Geometry: final body of the model. Coordinates: model frame, mm. Give positions to 0.01 mm unless a question says otherwise; leave off trailing zeros. Order: outer loops, then holes, each group sorted by start corner. A loop starts at its lowest first (then second) coordinate and runs counter-clockwise, first axis right, second up. Notation, with made-up numbers: M 21.25,72.5 L 78.25,72.5 A34 ccw 78.25,111.5 Z; hole C 48.25,-34 d6. An arc over 180 degrees is marked long. Write item = value, one per line. Start each with the question number.
from build123d import *

# Parameters (mm, degrees)
F1_ANGLE    = 180
F2_R        = 3.75
F3_DEPTH    = 5
F4_T4_ANGLE = 81.9757587875


# Not quite as in the source:
# - a fillet or chamfer that OpenCascade refuses, or shapes differently, is made with other operations: its cross-section is extruded or revolved along the edge and cut away or added
# - a feature names something its author has since deleted; it is built from what else it names


with BuildPart() as f1:
    # F0 (on Top) → F1 (revolve)
    with BuildSketch(Plane.XY):
        with BuildLine():
            ThreePointArc((-26, 0), (0, 26), (26, 0))
            Line((26, 0), (28.5, 0))
            ThreePointArc((28.5, 0), (0, 28.5), (-28.5, 0))
            Line((-28.5, 0), (-26, 0))
        make_face()
    revolve(axis=Axis((0, 0, 0), (1, 0, 0)), revolution_arc=F1_ANGLE)

    # F2 (on Top) → F3 (join)
    with BuildSketch(Plane.XY):
        with BuildLine():
            Line((64.7386337537, 8), (24.7386337537, 8))
            ThreePointArc((24.7386337537, 8), (25.6827225737, 4.0494149209), (26, 0))
            ThreePointArc((26, 0), (25.6827225737, -4.0494149209), (24.7386337537, -8))
            Line((24.7386337537, -8), (66.83281573, -8))
            ThreePointArc((66.83281573, -8), (72.8068677326, 0.918971944), (64.7386337537, 8))
        make_face()
        with Locations((64.7386337537, -0.1370499422)):
            Circle(F2_R, mode=Mode.SUBTRACT)
    extrude(amount=F3_DEPTH)

    # F4: chamfer of 5 on 1 edges, made by hand


with BuildPart() as f4_tool2:
    # F4_s3 → F4_t4 (revolve)
    with BuildSketch(Plane(origin=(0, 0, 0), x_dir=(0, 0, 1), z_dir=(-0.6558993597, -0.754848349, 0))):
        with BuildLine():
            Line((4.8832304356, -32.8400371197), (9.1867076398, -26.8558845985))
            Line((9.1867076398, -26.8558845985), (9.1548832957, -26.761083696))
            ThreePointArc((9.1548832957, -26.761083696), (7.1037600734, -27.4972106371), (4.9824561404, -27.9595266557))
            Line((4.9824561404, -27.9595266557), (4.9, -28.0579756932))
            ThreePointArc((4.9, -28.0579756932), (4.9, -30.4490064064), (4.7832304356, -32.8400371197))
            Line((4.7832304356, -32.8400371197), (4.8832304356, -32.8400371197))
        make_face()
    revolve(axis=Axis((0, 0, 5), (0, 0, 1)), revolution_arc=F4_T4_ANGLE)

    split(bisect_by=Plane.XZ.offset(8), keep=Keep.BOTTOM)

    split(bisect_by=Plane.XZ.offset(-8), keep=Keep.TOP)


with BuildPart() as f1_1:
    add(f1.part)

    # F4_t1: union F4_tool2
    add(f4_tool2.part)


solid = f1_1.part
1) Cut plane A-A (z = 2.25). Return loops of the section in (x, y).
2) Pin query (flat end, axial travel): pin 1 Ø10 at (y, z) = (-5.5, 24.5) entering from -X; pin 2 Ø4.5 at (x, z) = (47, 3) entering from +Y; pin 3 Ø12 at (x, y) = (-10.5, 6.5) entering from +Z. Return the tip coordinate at first contact, or that it passes through.
3) Cut plane B-B (x = 58.5). Return loops of the section in (y, z), plus the area to 3 significant figures.
4) Cut plane D-D (y = -18). Return loops of the section in (x, z), plus the area to 3 significant figures.
5) Cut plane C-C (z = 16.25). Return loops of the section in (x, y), plus the area to 3 significant figures.
6) Draft query along Y for faces 1 (the cylindrical face through (68.203, -1.573, 2.465)), 2 (the flat face through (46, 8, 2)), 3 (the cylindrical face through (72.827, 0.756, 2.465)). Return one class per face: pulls with the +Y half, pulls with the -Y half, needs draft (parallel to the pull), parting line crosses it, or undercut.
7) Ray query, L1, parallel to Y at x = 27, z = 8; L2, parallel to Z at x = 59, y = -3; L3, parallel to X at y = -8.5, z = 1.5. Return the intervals inside material, ascending.
Reply:
q1.outline = M 27.26,-8 L 66.83,-8 A8.14 ccw 64.74,8 L 27.26,8 A28.41 ccw long Z; hole C 0,0 d51.8; hole C 64.74,-0.14 d7.5
q2.pin_1 = -20.2
q2.pin_2 = 8
q2.pin_3 = 27.78
q3.outline = M -8,0 L 8,0 L 8,5 L -8,5 Z
q3.area = 80.0 mm²
q4.outline = M -22.1,0 L -18.76,0 A18.76 cw 18.76,0 L 22.1,0 A22.1 ccw Z
q4.area = 214 mm²
q5.outline = C 0,0 d46.83; hole C 0,0 d40.59
q5.area = 428 mm²
q6.face_1 = undercut
q6.face_2 = pulls with the +Y half
q6.face_3 = parting line crosses it
q7.L1 = -8 to 8
q7.L2 = 0 to 5
q7.L3 = -27.16 to -24.53, 24.53 to 27.16
